```python
from build123d import *

# Parameters (mm, degrees)
SKETCH1_R           = 6
BOSS_EXTRUDE1_DEPTH = 150
SKETCH2_OUTSIDE_W   = 44.192
SKETCH2_OUTSIDE_H   = 44.192
SKETCH2_OUTSIDE_R   = 4
CUT_EXTRUDE1_DEPTH  = 26
SKETCH3_OUTSIDE_W   = 44.192
SKETCH3_OUTSIDE_H   = 44.192
SKETCH3_OUTSIDE_R   = 4
CUT_EXTRUDE2_DEPTH  = 42
SKETCH4_W           = 0.5
SKETCH4_H           = 32
CUT_EXTRUDE3_DEPTH  = 5
CHAMFER1_SIZE       = 0.5


with BuildPart() as part:
    # Sketch1 → Boss-Extrude1 (new body)
    with BuildSketch(Plane(origin=(0, 0, 0), x_dir=(1, 0, 0), z_dir=(0, 1, 0))):
        with Locations(Location((0, 0, 0), (0, 0, 270))):
            Circle(SKETCH1_R)
    extrude(amount=BOSS_EXTRUDE1_DEPTH)

    # Sketch2 outside → Cut-Extrude1 (cut)
    with BuildSketch(Plane(origin=(0, 150, 0), x_dir=(1, 0, 0), z_dir=(0, 1, 0))):
        Rectangle(SKETCH2_OUTSIDE_W, SKETCH2_OUTSIDE_H)
        with Locations(Location((0, 0, 0), (0, 0, 270))):
            Circle(SKETCH2_OUTSIDE_R, mode=Mode.SUBTRACT)
    extrude(amount=-CUT_EXTRUDE1_DEPTH, mode=Mode.SUBTRACT)

    # Sketch3 outside → Cut-Extrude2 (cut)
    with BuildSketch(Plane.XZ):
        Rectangle(SKETCH3_OUTSIDE_W, SKETCH3_OUTSIDE_H)
        with Locations(Location((0, 0, 0), (0, 0, 90))):
            Circle(SKETCH3_OUTSIDE_R, mode=Mode.SUBTRACT)
    extrude(amount=-CUT_EXTRUDE2_DEPTH, mode=Mode.SUBTRACT)

    # Sketch4 → Cut-Extrude3 (cut, symmetric)
    with BuildSketch(Plane(origin=(0, 0, 0), x_dir=(0, 0, -1), z_dir=(1, 0, 0))):
        with Locations((-3.75, 16)):
            Rectangle(SKETCH4_W, SKETCH4_H)
    extrude(amount=CUT_EXTRUDE3_DEPTH, both=True, mode=Mode.SUBTRACT)

    # Chamfer1
    chamfer1_edges = [part.edges().sort_by_distance(p)[0] for p in [
        (0, 0, -4),
        (0, 150, -4),
    ]]
    chamfer(chamfer1_edges, length=CHAMFER1_SIZE - 0.0001)  # a hair under: the kernel refuses the full size


solid = part.part
```
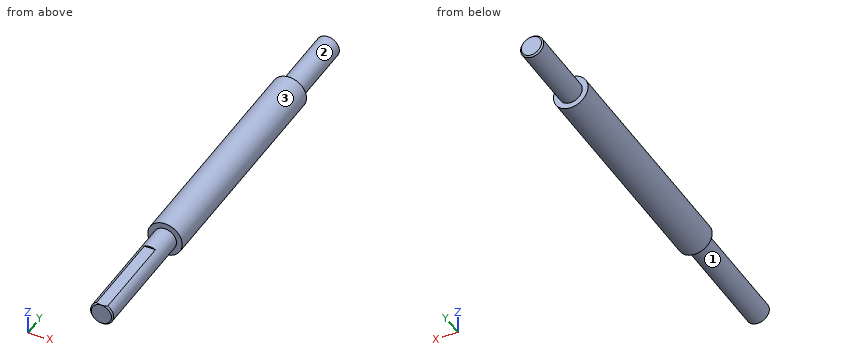
CAD build for the part. Positions are in the model's coordinates, mm. Face numbers are marked on the shaded views. A direction names the side the tool comes from. Round coordinates to 2 decimals unless told otherwise and drop trailing zeros. Order: outer loops, then holes, each group sorted by start corner. A loop starts at its lowest first (then second) coordinate and runs counter-clockwise, first axis right, second up.
Item 1: Probe line 1 along Y through (x, z) = (-4.75, 0.75); line 2 along Z through (x, y) = (-1.5, 97.5); line 3 along X through (y, z) = (138.5, 2.25). List the from-to ranges inside material, lowest first.
Item 2: Saw through at B-B on y = 52.5. Write the cut outline in (x, z).
Item 3: Tool access for the marked faces 1, 2 and 3: list every direction of +Z, -Z, +X, -X, +Y, -Y with a clear straight run to the whole face (end or side of a thin tool).
Item 4: Saw through at A-A on z = 0. Write the cut outline in (x, y).
Item 5: Pin check, flat tips, straight feed: pin 1 (3.5 mm diameter, centred on x = 1.5, z = 1, fed in from -Y); pin 2 (6 mm diameter, centred on y = 133.5, z = -3, fed in from -X); pin 3 (1.2 mm diameter, centred on x = 0.5, y = 19.5, fed in from +Z). Stop position of each tip, or through.
Reported:
1. line 1: y = 42 to 124
1. line 2: z = -5.81 to 5.81
1. line 3: x = -3.31 to 3.31
2. outline: circle Ø12 at (0, 0)
3. face 1: -Y
3. face 2: +Y
3. face 3: +Y, -Y
4. outline: (-6, 42) - (-4, 42) - (-4, 0.5) - (-3.5, 0) - (3.5, 0) - (4, 0.5) - (4, 42) - (6, 42) - (6, 124) - (4, 124) - (4, 149.5) - (3.5, 150) - (-3.5, 150) - (-4, 149.5) - (-4, 124) - (-6, 124) - close
5. pin 1: stops at y = 0
5. pin 2: stops at x = -4
5. pin 3: stops at z = 3.5
